Design review of the part built by this model. Coordinates are the model's own, in mm. Round coordinates to 2 decimals unless told otherwise and drop trailing zeros. Loops run counter-clockwise (first coordinate to the right, second up) from the corner with the lowest first, then second, coordinate; pieces in that order, holes last. Notation, with made-up numbers: (53.25, 15) -> (92.25, 15) arc R15 cw to (92.25, 43) -> close; hole circle Ø3 at (56.5, 6.25). An arc over 180 degrees is marked (long way). Write each question's results on one line, items separated by ' | '. Start each with the question number.
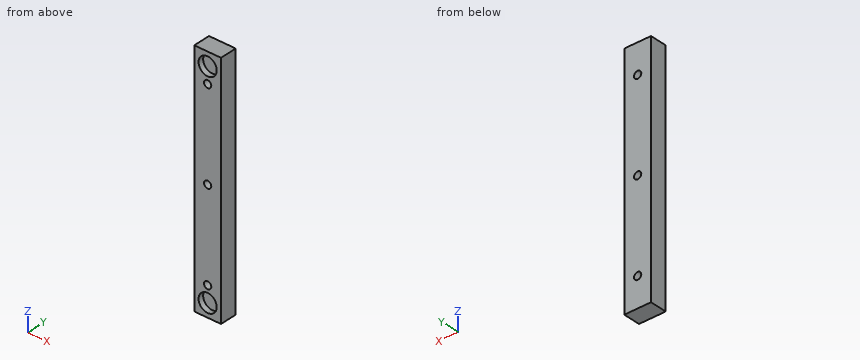
from build123d import *

# Parameters (mm, degrees)
SKETCH1_W           = 25
SKETCH1_H           = 225
BOSS_EXTRUDE1_DEPTH = 16
SKETCH2_R           = 8.5
CUT_EXTRUDE1_DEPTH  = 5
M8_TAPPED_HOLE1_D   = 6.8


with BuildPart() as part:
    # Sketch1 → Boss-Extrude1 (new body)
    with BuildSketch(Plane(origin=(0, 0, 0), x_dir=(1, 0, 0), z_dir=(0, 1, 0))):
        Rectangle(SKETCH1_W, SKETCH1_H)
    extrude(amount=-BOSS_EXTRUDE1_DEPTH)

    # Sketch2 → Cut-Extrude1 (cut)
    with BuildSketch(Plane.XZ.offset(16)):
        with Locations(Location((0, 100, 0), (0, 0, 270))):
            Circle(SKETCH2_R)
        with Locations(Location((0, -100, 0), (0, 0, 270))):
            Circle(SKETCH2_R)
    extrude(amount=-CUT_EXTRUDE1_DEPTH, mode=Mode.SUBTRACT)

    # M8 Tapped Hole1 (through all)
    with Locations(Plane(origin=(0, 0, 0), x_dir=(1, 0, 0), z_dir=(0, 1, 0))):
        with Locations((0, 85), (0, 0), (0, -85)):
            Hole(M8_TAPPED_HOLE1_D / 2)


solid = part.part
1) To check wall thickness, follow line 1 (Z direction, x = 0, y = -8.75); line 2 (X direction, y = -12.5, z = -85); line 3 (Z direction, x = 2.25, y = -11.5). State the ranges of each line that lie inside material, in increasing order. Write a range as from..to.
2) Take a section at C-C (y = -8). Write out the cut boundary in (x, z), plus the area to 3 significant figures.
3) Take a section at D-D (z = -100). Write out the cut boundary in (x, y).
4) Take a section at A-A (z = 0). Write out the cut boundary in (x, y).
5) Insertion check: pin 1 (5 mm diameter, centred on x = -3.5, z = 101.5, fed in from -Y). The pin has a flat end and moves straight along its axis. Give the tip position at first contact, or say it passes through.
6) Take a section at B-B (x = 0). Write out the cut boundary in (y, z).
Geometry check:
1) line 1: z = -112.5..-88.4, -81.6..-3.4, 3.4..81.6, 88.4..112.5 | line 2: x = -12.5..-3.4, 3.4..12.5 | line 3: z = -112.5..-108.2, -91.8..-87.55, -82.45..-2.55, 2.55..82.45, 87.55..91.8, 108.2..112.5
2) outline: (-12.5, -112.5) -> (12.5, -112.5) -> (12.5, 112.5) -> (-12.5, 112.5) -> close; hole circle Ø6.8 at (0, -85); hole circle Ø6.8 at (0, 0); hole circle Ø6.8 at (0, 85) | area: 5,520 mm^2
3) outline: (-12.5, -16) -> (-8.5, -16) -> (-8.5, -11) -> (8.5, -11) -> (8.5, -16) -> (12.5, -16) -> (12.5, 0) -> (-12.5, 0) -> close
4) outline: (-12.5, -16) -> (-3.4, -16) -> (-3.4, 0) -> (-12.5, 0) -> close; (3.4, -16) -> (12.5, -16) -> (12.5, 0) -> (3.4, 0) -> close
5) pin 1: stops at y = -11
6) outline: (-16, -112.5) -> (0, -112.5) -> (0, -88.4) -> (-16, -88.4) -> (-16, -91.5) -> (-11, -91.5) -> (-11, -108.5) -> (-16, -108.5) -> close; (-16, -81.6) -> (0, -81.6) -> (0, -3.4) -> (-16, -3.4) -> close; (-16, 3.4) -> (0, 3.4) -> (0, 81.6) -> (-16, 81.6) -> close; (-16, 88.4) -> (0, 88.4) -> (0, 112.5) -> (-16, 112.5) -> (-16, 108.5) -> (-11, 108.5) -> (-11, 91.5) -> (-16, 91.5) -> close
